Part model, mm, in its own coordinate system. Face numbers are marked on the shaded views. A direction names the side the tool comes from. Round coordinates to 2 decimals unless told otherwise and drop trailing zeros. Write each loop counter-clockwise with the first axis right and the second up, starting at its lowest first coordinate (ties: lowest second). Pieces come first, ordered by that corner, then holes. Notation, with made-up numbers: M -33,23.25 L -15,23.25 A31 ccw -15,58.25 Z; hole C 32.25,29.5 d10. An arc over 180 degrees is marked long. One line per question, with ' | ' between items. Start each with the question number.
1) Saw through at A-A (y = -7). List the corners of the cut face in (x, z), plus the area to 3 significant figures.
2) Saw through at D-D (x = -12). List the corners of the cut face in (y, z), plus the area to 3 significant figures.
3) Wall check: probe 1 along Y at (x, z) = (-16, 3); probe 2 along Z at (x, y) = (0, -3.5); probe 3 along X at (y, z) = (-7.5, 11.5). Give the ranges that are in metal, low to high. Write a range as [from, to].
4) Mould opens along X. For the marked faces 1, 2, 3 and 4 say: pulls with the +X half, pulls with the -X half, needs draft (parallel to the pull), parting line crosses it, or undercut.
5) Drop flat-ended pins along their axis: pin 1 Ø4 at (y, z) = (-11, 28.5) entering from -X; pin 2 Ø3 at (x, y) = (-16.04, -7) entering from -Z; pin 3 Ø6 at (x, y) = (13.5, -4.5) entering from +Z; pin 4 Ø8 at (x, y) = (-13, -3) entering from -Z. Give the stop position or say it passes through.
6) Saw through at B-B (z = 20). List the corners of the cut face in (x, y), plus the area to 3 significant figures.
7) Tool access for the marked faces 5, 6 and 7: list every direction of +Z, -Z, +X, -X, +Y, -Y with a clear straight run to the whole face (end or side of a thin tool).
8) Saw through at C-C (y = -3). List the corners of the cut face in (x, z).
```python
from build123d import *

# Parameters (mm, degrees)
F0_W     = 12
F0_H     = 6
F0_R     = 4
F1_DEPTH = 14
F3_D     = 5
F3_DEPTH = 6
F3_TIP   = 1.5021515476


with BuildPart() as f1:
    # F0 (on Front) → F1 (new body)
    with BuildSketch(Plane.XZ):
        with Locations((-15, 3)):
            Rectangle(F0_W, F0_H)
        Polygon((-9, 0), (0, 0), (9, 0), (9, 6), (9, 32.8), (0, 32.8), (-9, 32.8), (-9, 6), align=None)
        with Locations((0, 20)):
            Circle(F0_R, mode=Mode.SUBTRACT)
        with Locations((15, 3)):
            Rectangle(F0_W, F0_H)
    extrude(amount=F1_DEPTH)

    # F3
    with Locations(Plane(origin=(0, 0, 0), x_dir=(1, 0, 0), z_dir=(0, 0, -1))):
        with Locations((-16.037677303, 7), (15.962322697, 7)):
            Hole(F3_D / 2, depth=F3_DEPTH)
            with Locations((0, 0, -(F3_DEPTH + F3_TIP / 2))):  # 118° drill point
                Cone(0, F3_D / 2, F3_TIP, mode=Mode.SUBTRACT)


solid = f1.part
```
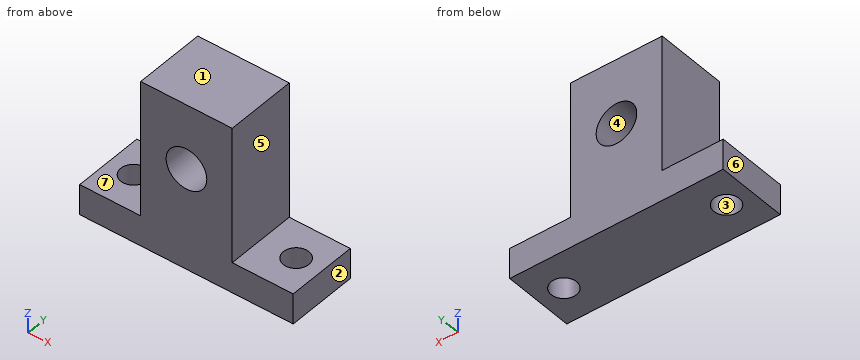
Answer key:
1) outline: M -21,0 L -18.54,0 L -18.54,6 L -21,6 Z; M -13.54,0 L 13.46,0 L 13.46,6 L 9,6 L 9,32.8 L -9,32.8 L -9,6 L -13.54,6 Z; M 18.46,0 L 21,0 L 21,6 L 18.46,6 Z; hole C 0,20 d8 | area: 624 mm2
2) outline: M -14,0 L 0,0 L 0,6 L -14,6 Z | area: 84.0 mm2
3) probe 1: y = [-14, -9.5], [-4.5, 0] | probe 2: z = [0, 16], [24, 32.8] | probe 3: x = [-9, 9]
4) face 1: needs draft | face 2: pulls with the +X half | face 3: undercut | face 4: undercut
5) pin 1: stops at x = -9 | pin 2: passes through | pin 3: stops at z = 6 | pin 4: stops at z = 0
6) outline: M -9,-14 L -4,-14 L -4,0 L -9,0 Z; M 4,-14 L 9,-14 L 9,0 L 4,0 Z | area: 140 mm2
7) face 5: +Z, +X, +Y, -Y | face 6: +Z, -Z, -X, +Y, -Y | face 7: +Z, -X, +Y, -Y
8) outline: M -21,0 L 21,0 L 21,6 L 9,6 L 9,32.8 L -9,32.8 L -9,6 L -21,6 Z; hole C 0,20 d8
